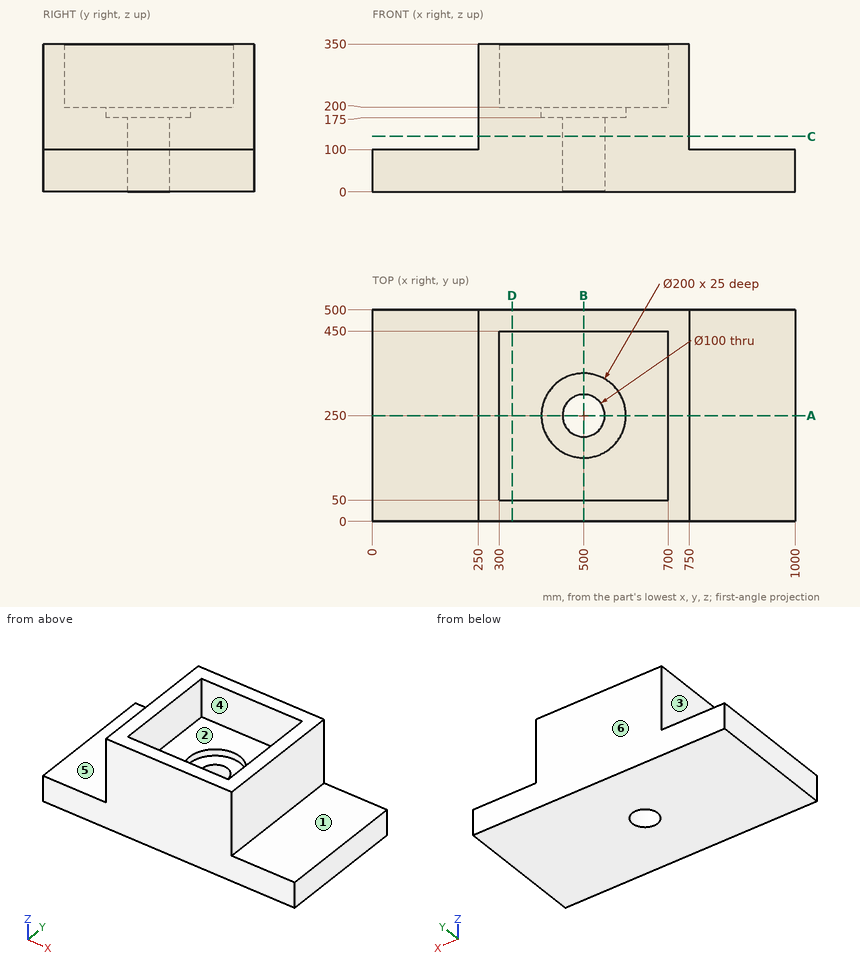
The drawing under review shows one solid part. Ordinate dimensions are in mm from its lowest x, y, z. A direction names the side the tool comes from. Coordinates: 2 decimals unless noted, no trailing zeros. Write each loop counter-clockwise with the first axis right and the second up, starting at its lowest first coordinate (ties: lowest second). Pieces come first, ordered by that corner, then holes. Notation, with made-up numbers: (-2.75, 0.5) - (8.25, 0.5) arc R17 cw to (8.25, 5.5) - close; hole circle Ø6 at (86.5, -26). An arc over 180 degrees is marked (long way). Answer in a Markdown table with one row per item. Add a question column.
Q1. We need section A-A, the plane y = 250. State the section outline as (x, z) points, and give its area (4 significant figures).
Q2. We need section C-C, the plane z = 131.5. State the section outline as (x, y) points, and give its area (3 significant figures).
Q3. We need section B-B, the plane x = 500. State the section outline as (y, z) points, and give its area (3 significant figures).
Q4. For probe 1 along Y at (x, z) = (500, 183); probe 2 along Y at (x, z) = (500, 43); probe 3 along X at (y, z) = (165.5, 298), list the stretches that pass through material, from the lowest coordinate up.
Q5. Tool access review of the marked faces 1, 2 and 3: name each direction out of +Z, -Z, +X, -X, +Y, -Y from which nothing blocks a thin tool from reaching the whole face with its end or side.
Q6. We need section D-D, the plane x = 330.5. State the section outline as (y, z) points, and give its area (3 significant figures).
Q7. For P1, Ø4, axis at y = 374.5, z = 284.5, coming from the +X side; P2, Ø5, axis at x = 283.5, z = 240, coming from the -Y side; P3, Ø8, axis at y = 168.5, z = 301, coming from the -X side, all flat-tipped, find the tip position at first contact; note any pin that passes through.
Q8. Draft analysis for pull direction Y (two halves, no side actions). For the marked faces 4, 5 and 6, state which applies: +Y half, -Y half, draft (parallel to the pull), parting line (faces both ways), or undercut.
Answer list:
| question | item | result |
|---|---|---|
| 1 | outline | (0, 0) - (450, 0) - (450, 175) - (400, 175) - (400, 200) - (300, 200) - (300, 350) - (250, 350) - (250, 100) - (0, 100) - close; (550, 0) - (1000, 0) - (1000, 100) - (750, 100) - (750, 350) - (700, 350) - (700, 200) - (600, 200) - (600, 175) - (550, 175) - close |
| 1 | area | 142,500 mm2 |
| 2 | outline | (250, 0) - (750, 0) - (750, 500) - (250, 500) - close; hole circle Ø100 at (500, 250) |
| 2 | area | 242,000 mm2 |
| 3 | outline | (0, 0) - (200, 0) - (200, 175) - (150, 175) - (150, 200) - (50, 200) - (50, 350) - (0, 350) - close; (300, 0) - (500, 0) - (500, 350) - (450, 350) - (450, 200) - (350, 200) - (350, 175) - (300, 175) - close |
| 3 | area | 92,500 mm2 |
| 4 | probe 1 | y = 0 to 150, 350 to 500 |
| 4 | probe 2 | y = 0 to 200, 300 to 500 |
| 4 | probe 3 | x = 250 to 300, 700 to 750 |
| 5 | face 1 | +Z, +X, +Y, -Y |
| 5 | face 2 | +Z |
| 5 | face 3 | +Z, -X, +Y, -Y |
| 6 | outline | (0, 0) - (500, 0) - (500, 350) - (450, 350) - (450, 200) - (50, 200) - (50, 350) - (0, 350) - close |
| 6 | area | 115,000 mm2 |
| 7 | P1 | stops at x = 750 |
| 7 | P2 | stops at y = 0 |
| 7 | P3 | stops at x = 250 |
| 8 | face 4 | undercut |
| 8 | face 5 | draft |
| 8 | face 6 | +Y half |
